from build123d import *

# Parameters (mm, degrees)
SKETCH1_W                    = 1206.5
SKETCH1_H                    = 596.9
BOSS_EXTRUDE1_DEPTH          = 17.78
F_1_8_0_125_DIAMETER_HOLE1_D = 3.175
FILLET1_R                    = 6.35
SKETCH4_W                    = 158.75
SKETCH4_H                    = 152.4
SKETCH4_W_2                  = 152.4
CUT_EXTRUDE1_DEPTH           = 12.7
FILLET2_R                    = 6.35


with BuildPart() as part:
    # Sketch1 → Boss-Extrude1 (new body)
    with BuildSketch(Plane(origin=(0, 0, 0), x_dir=(1, 0, 0), z_dir=(0, 1, 0))):
        Rectangle(SKETCH1_W, SKETCH1_H)
    extrude(amount=BOSS_EXTRUDE1_DEPTH)

    # 1/8 (0.125) Diameter Hole1 (through all)
    with Locations(Plane(origin=(0, 17.78, 0), x_dir=(1, 0, 0), z_dir=(0, 1, 0))):
        with Locations((0, 0), (457.2, 152.4), (-457.2, -152.4), (-457.2, 152.4), (457.2, -152.4)):
            Hole(F_1_8_0_125_DIAMETER_HOLE1_D / 2)

    # Fillet1
    fillet1_edges = [part.edges().sort_by_distance(p)[0] for p in [
        (603.25, 8.89, 298.45),
        (-603.25, 8.89, 298.45),
        (-603.25, 8.89, -298.45),
        (603.25, 8.89, -298.45),
    ]]
    fillet(fillet1_edges, radius=FILLET1_R)

    # Sketch4 → Cut-Extrude1 (cut)
    with BuildSketch(Plane(origin=(0, 17.78, 0), x_dir=(1, 0, 0), z_dir=(0, 1, 0))):
        with Locations((0, -222.25)):
            Rectangle(SKETCH4_W, SKETCH4_H)
        with Locations((-527.05, 0)):
            Rectangle(SKETCH4_W_2, SKETCH4_H)
    extrude(amount=-CUT_EXTRUDE1_DEPTH, mode=Mode.SUBTRACT)

    # Fillet2
    fillet2_edges = [part.edges().sort_by_distance(p)[0] for p in [
        (79.375, 11.43, 146.05),
        (79.375, 11.43, 298.45),
        (-79.375, 11.43, 298.45),
        (-79.375, 11.43, 146.05),
        (-603.25, 11.43, 76.2),
        (-603.25, 11.43, -76.2),
        (-450.85, 11.43, -76.2),
        (-450.85, 11.43, 76.2),
    ]]
    fillet(fillet2_edges, radius=FILLET2_R)


solid = part.part
Source: CAD feature listing. Evaluate the final solid. Frame: model axes, mm. A direction names the side the tool comes from. Coordinates: 2 decimals unless noted, no trailing zeros. Loops run counter-clockwise (first coordinate to the right, second up) from the corner with the lowest first, then second, coordinate; pieces in that order, holes last. Notation, with made-up numbers: (79, 87.25) - (91, 87.25) arc R27 ccw to (91, 118.25) - close; hole circle Ø3 at (84, 59). An arc over 180 degrees is marked (long way). One line per item, written item: value. Start each with the question number.
1. Contact query for flat-ended pins moving along their axis: P1, Ø12, axis at x = 350, z = 99, coming from the -Y side; P2, Ø1.9, axis at x = 0, z = 0, coming from the +Y side; P3, Ø5, axis at y = 14.5, z = 23, coming from the -X side. Output: stop coordinate, or through.
2. Mould query, pull axis Z, two halves, no side actions, for faces 3 (the flat face through (-528, 5.08, -1)), 4 (the flat face through (-8, 0, -4)). Classes: pulls with the +Z half, pulls with the -Z half, needs draft (parallel to the pull), parting line crosses it, or undercut.
3. Section B-B (z = 217). Return the cut outline in (x, y) (3 decimals).
4. Section C-C (x = 14). Return the cut outline in (y, z).
5. Section A-A (y = 12.5). State how many separate pieces and enclosed holes the cut face has, and give its area (3 significant figures).
6. Set-up query: faces 1 (the flat face through (-8, 17.78, -4)), 2 (the flat face through (-1, 5.08, 221)). Return all of +Z, -Z, +X, -X, +Y, -Y with unobstructed straight access to the full face (end or side cutting, diameter ignored); none if empty.
7. Ray query, L1, parallel to Z at x = 457.2, y = 11.5; L2, parallel to Z at x = -487.5, y = 7.5; L3, parallel to X at y = 11, z = 243 (3 decimals). Return the intervals inside material, ascending.
Verdict:
1. P1: stops at y = 0
1. P2: passes through
1. P3: stops at x = -450.85
2. face 3: undercut
2. face 4: needs draft
3. outline: (-603.25, 0) - (603.25, 0) - (603.25, 17.78) - (79.375, 17.78) - (79.375, 5.08) - (-79.375, 5.08) - (-79.375, 17.78) - (-603.25, 17.78) - close
4. outline: (0, -298.45) - (17.78, -298.45) - (17.78, 146.05) - (5.08, 146.05) - (5.08, 298.45) - (0, 298.45) - close
5. separate pieces: 1
5. enclosed holes: 5
5. area: 673,000 mm2
6. face 1: +Z, -Z, +X, -X, +Y
6. face 2: +Z, +Y
7. L1: z = -298.45 to -153.99, -150.81 to 150.81, 153.99 to 298.45
7. L2: z = -298.45 to -76.2, 76.2 to 298.45
7. L3: x = -603.25 to -79.375, 79.375 to 603.25
